Source: CAD feature listing. Evaluate the final solid. Frame: model axes, mm. A direction names the side the tool comes from. Give positions to 0.01 mm unless a question says otherwise; leave off trailing zeros. Order: outer loops, then holes, each group sorted by start corner. A loop starts at its lowest first (then second) coordinate and runs counter-clockwise, first axis right, second up. Notation, with made-up numbers: (-9.5, -5.5) - (37.5, -5.5) arc R8 ccw to (37.5, 2.5) - close; hole circle Ø3 at (79.5, 33). An arc over 180 degrees is marked (long way). Answer as CSV lines item,"result".
```python
from build123d import *

# Parameters (mm, degrees)
SKETCH2_W           = 35
SKETCH2_H           = 24
BOSS_EXTRUDE1_DEPTH = 10
SKETCH3_R           = 6
BOSS_EXTRUDE2_DEPTH = 12
SKETCH4_R           = 5
CUT_EXTRUDE2_DEPTH  = 2


with BuildPart() as part:
    # Sketch2 → Boss-Extrude1 (new body)
    with BuildSketch(Plane(origin=(0, 0, 0), x_dir=(1, 0, 0), z_dir=(0, 1, 0))):
        Rectangle(SKETCH2_W, SKETCH2_H)
    extrude(amount=BOSS_EXTRUDE1_DEPTH)

    # Sketch3 → Boss-Extrude2 (add)
    with BuildSketch(Plane(origin=(0, 10, 0), x_dir=(1, 0, 0), z_dir=(0, 1, 0))):
        with Locations((8.5, 0)):
            Circle(SKETCH3_R)
    extrude(amount=BOSS_EXTRUDE2_DEPTH)

    # Sketch4 → Cut-Extrude2 (cut)
    with BuildSketch(Plane(origin=(0, 22, 0), x_dir=(1, 0, 0), z_dir=(0, 1, 0))):
        with Locations((8.5, 0)):
            Circle(SKETCH4_R)
    extrude(amount=-CUT_EXTRUDE2_DEPTH, mode=Mode.SUBTRACT)


solid = part.part
```
(1) Contact query for flat-ended pins moving along their axis: pin 1 (5 mm diameter, centred on x = 10, z = 0, fed in from +Y); pin 2 (8 mm diameter, centred on y = 16.5, z = 8.5, fed in from +X); pin 3 (1 mm diameter, centred on x = 1.5, z = 4, fed in from +Y). Output: stop coordinate, or through.
Completed:
pin 1,"y = 20"
pin 2,"x = 12.47"
pin 3,"y = 10"
(2) Access query for faces 1 (the cylindrical face through (13.27, 21.01, -1.5)), 2 (the flat face through (7, 22, -5)). Directions: +Z, -Z, +X, -X, +Y, -Y. A direction counts if a zero-diameter tool reaches every point of the face in a straight line with its end or side. Return the directions, or none.
Completed:
face 1,"+Y"
face 2,"+Z, -Z, +X, -X, +Y"
(3) Cut plane A-A (z = 0). Return loops of the section in (x, y), then the cut area to 3 significant figures.
Completed:
outline,"(-17.5, 0) - (17.5, 0) - (17.5, 10) - (14.5, 10) - (14.5, 22) - (13.5, 22) - (13.5, 20) - (3.5, 20) - (3.5, 22) - (2.5, 22) - (2.5, 10) - (-17.5, 10) - close"
area,"474 mm²"
(4) Cut plane C-C (y = 15.75). Return loops of the section in (x, z), then the cut area to 3 significant figures.
Completed:
outline,"circle Ø12 at (8.5, 0)"
area,"113 mm²"
(5) Ray query, line 1 (Z direction, x = 8.5, y = 20.75); line 2 (X direction, y = 21, z = 0); line 3 (Y direction, x = -8.5, z = 7.25). Return the intervals inside material, ascending. Write a range as from..to.
Completed:
line 1,"-6..-5, 5..6"
line 2,"2.5..3.5, 13.5..14.5"
line 3,"0..10"
(6) Cut plane D-D (x = 3). Return loops of the section in (y, z), then the cut area to 3 significant figures.
Completed:
outline,"(0, -12) - (10, -12) - (10, -2.4) - (22, -2.4) - (22, 2.4) - (10, 2.4) - (10, 12) - (0, 12) - close"
area,"298 mm²"
(7) Mould query, pull axis X, two halves, no side actions, for faces 3 (the flat face through (8, 20, 0)), 4 (the flat face through (17.5, 5, 0)), 5 (the flat face through (-17.5, 5, 0)), 6 (the flat face through (0, 5, -12)). Classes: released by +X, released by -X, zero draft, split by the parting line, or undercut.
Completed:
face 3,"undercut"
face 4,"released by +X"
face 5,"released by -X"
face 6,"zero draft"
(8) Cut plane B-B (x = 8.5). Return loops of the section in (y, z), then the cut area to 3 significant figures.
Completed:
outline,"(0, -12) - (10, -12) - (10, -6) - (22, -6) - (22, -5) - (20, -5) - (20, 5) - (22, 5) - (22, 6) - (10, 6) - (10, 12) - (0, 12) - close"
area,"364 mm²"
